```python
from build123d import *

# Parameters (mm, degrees)
F2_R      = 37.5
F3_DEPTH  = 4
F5_R      = 30
F6_DEPTH  = 12
F8_R      = 37.5
F9_DEPTH  = 4
F15_R     = 3.5296355076
F16_DEPTH = 5


with BuildPart() as f3:
    # F2 (on Top) → F3 (new body)
    with BuildSketch(Plane.XY):
        Circle(F2_R)
    extrude(amount=F3_DEPTH)

    # F5 (on offset) → F6 (join)
    with BuildSketch(Plane.XY.offset(4)):
        Circle(F5_R)
    extrude(amount=F6_DEPTH)

    # F8 (on offset) → F9 (join)
    with BuildSketch(Plane.XY.offset(16)):
        Circle(F8_R)
    extrude(amount=F9_DEPTH)


with BuildPart() as f10_1:
    # F10: copy of F3
    add(f3.part.moved(Location((0, 0, 20))))


with BuildPart() as f12_1:
    # F12: copy of F3
    add(f3.part)


with BuildPart() as f3_1:
    # F14: moved
    add(f3.part.moved(Location((0, 0, 40))))

    # F15 (on face) → F16 (join)
    with BuildSketch(Plane.XY.offset(60)):
        with Locations((-18.8314225525, 23.8138604909)):
            Circle(F15_R)
    extrude(amount=F16_DEPTH)


solid = f3_1.part
```
Here's how the part is built. I have some questions about the finished solid (model axes, mm). A direction names the side the tool comes from. Coordinates: 2 decimals unless noted, no trailing zeros. Order: outer loops, then holes, each group sorted by start corner. A loop starts at its lowest first (then second) coordinate and runs counter-clockwise, first axis right, second up. Notation, with made-up numbers: M 15.25,-14 L 51.25,-14 A21 ccw 51.25,-10 Z; hole C 56,39.5 d7. An arc over 180 degrees is marked long. Answer as a JSON object with one key per item and string values. Group by question number.
(1) For pin 1 (12 mm diameter, centred on x = -8.5, z = 52.5, fed in from -Y); pin 2 (3 mm diameter, centred on y = 14, z = 53.5, fed in from -X); pin 3 (2 mm diameter, centred on x = 13, y = 2, fed in from +Z), each with a flat end and sliding along its axis, tell me the tip position at first contact or that it passes through.
(2) I need wall thicknesses on probe 1 along Z at (x, y) = (30, 5); probe 2 along Z at (x, y) = (12, -2); probe 3 along X at (y, z) = (12, 46). Which ranges of each line are inside material? Lowest first, please.
(3) Suppose I cut it at D-D, the plane x = -19. Please give me the cut outline in (y, z).
(4) Suppose I cut it at A-A, the plane x = 0. Please give me the cut outline in (y, z), then the cut area to 3 significant figures.
(5) If we mould it in two halves opening along Z, with no side actions, what happens to faces 3 (the face through (-17, 25, 56)), 4 (the face through (-19, 24, 65)), 5 (the face through (-19.291, 27.313, 62.465))? For each: released by +Z, released by -Z, zero draft, split by the parting line, or undercut.
(6) Which directions (+Z, -Z, +X, -X, +Y, -Y) give clear straight access to the entire face, cutting with the end or side of a thin tool? Please do faces 1 (the face through (-1, 1, 40)), 2 (the face through (-29.97, 1.32, 49.92)).
(7) Suppose I cut it at C-C, the plane z = 53.75. Please give me the cut outline in (x, y).
Values found:
{
 "1": {"pin 1": "stops at y = -37.32", "pin 2": "stops at x = -27.27", "pin 3": "stops at z = 60"},
 "2": {"probe 1": "z = 40 to 44, 56 to 60", "probe 2": "z = 40 to 60", "probe 3": "x = -27.5 to 27.5"},
 "3": {"outline": "M -32.33,40 L 32.33,40 L 32.33,44 L 23.22,44 L 23.22,56 L 32.33,56 L 32.33,60 L 27.34,60 L 27.34,65 L 20.29,65 L 20.29,60 L -32.33,60 L -32.33,56 L -23.22,56 L -23.22,44 L -32.33,44 Z"},
 "4": {"outline": "M -37.5,40 L 37.5,40 L 37.5,44 L 30,44 L 30,56 L 37.5,56 L 37.5,60 L -37.5,60 L -37.5,56 L -30,56 L -30,44 L -37.5,44 Z", "area": "1,320 mm^2"},
 "5": {"face 3": "undercut", "face 4": "released by +Z", "face 5": "zero draft"},
 "6": {"face 1": "-Z, +X, -X, +Y, -Y", "face 2": "none"},
 "7": {"outline": "C 0,0 d60"}
}
